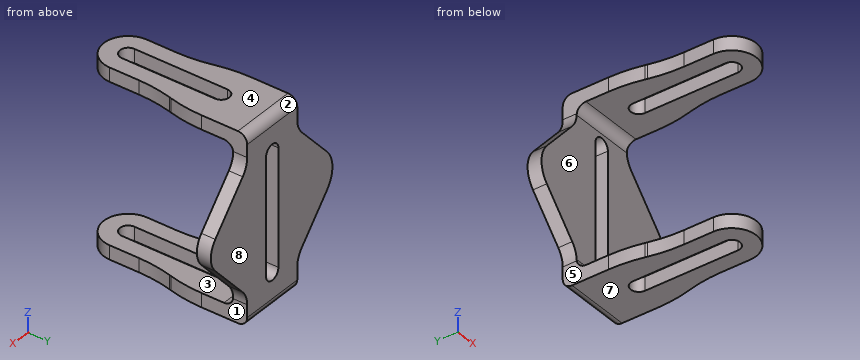
Autodesk Inventor part; units mm, degrees
ref_plane "YZ Plane" through (0, 0, 0) normal (1, 0, 0) x (0, 1, 0)
ref_plane "XZ Plane" through (0, 0, 0) normal (0, 1, 0) x (-1, 0, 0)
ref_plane "XY Plane" through (0, 0, 0) normal (0, 0, 1) x (1, 0, 0)
sketch "Sketch1" plane through (0, 0, 0) normal (0, 1, 0) x (-1, 0, 0)
  line L0 (7.1, -20.1) -> (-7.1, -20.1)
  line L1 (-7.1, -20.1) -> (-7.1, 20.1)
  line L2 (-7.1, 20.1) -> (7.1, 20.1)
  line L3 (7.1, 20.1) -> (7.1, -20.1)
  line L4 (7.1, -20.1) -> (-7.1, 20.1) construction
  line L5 (-7.1, -20.1) -> (7.1, 20.1) construction
  circle A0 centre (0, 12.1) radius 2
  point P0 (0, 0)
  dimension "d0" = 14.2
  dimension "d1" = 40.2
  dimension "d4" = 4
  dimension "d5" = 8
  dimension "d6" = 7.1
extrude "Extrusion1" add sketch "Sketch1" along normal blind 3 contours L0 L1 L2 L3 | A0
sketch "Sketch2" plane through (-7.1, 0, 20.1) normal (0, 0, 1) x (1, 0, 0)
  line L0 (7.1, -28) -> (7.1, -8) construction
  line L1 (8.85, -28) -> (8.85, -8)
  line L2 (5.35, -8) -> (5.35, -28)
  arc A0 (5.35, -28) -> (8.85, -28) centre (7.1, -28) ccw
  arc A1 (8.85, -8) -> (5.35, -8) centre (7.1, -8) ccw
  line L3 (0, 0) -> (0, 3)
  line L4 (0, 0) -> (14.2, 0)
  line L5 (1.85, -28) -> (1.85, -8)
  arc A2 (12.35, -8) -> (1.85, -8) centre (7.1, -8) ccw
  line L6 (12.35, -8) -> (12.35, -28)
  arc A3 (1.85, -28) -> (12.35, -28) centre (7.1, -28) ccw
  line L7 (0, 0) -> (0, -10.5)
  line L8 (0, -10.5) -> (1.85, -18)
  line L9 (14.2, 0) -> (14.2, -10.5)
  line L10 (14.2, -10.5) -> (12.35, -18)
  point P0 (7.1, 0)
  point P1 (7.1, -18)
  point P2 (8.85, -18)
  dimension "d7" = 7.1
  dimension "d8" = 3.5
  dimension "d9" = 20
  dimension "d10" = 18
  dimension "d11" = 3.5
extrude "Extrusion2" add sketch "Sketch2" against normal blind 3
mirror "Mirror1" about plane through (0, 0, 0) normal (0, 0, 1) of "Extrusion2"
fillet "Fillet1" radius 30 8 edges at (7.1, -10.5, 18.6) (5.25, -18, 18.6) (-7.1, -10.5, 18.6) (-5.25, -18, 18.6) (7.1, -10.5, -18.6) (5.25, -18, -18.6) (-7.1, -10.5, -18.6) (-5.25, -18, -18.6)
sketch "Sketch3" plane through (0, 3, 0) normal (0, 1, 0) x (1, 0, 0)
  line L0 (-7.1, -13.5) -> (7.1, -13.5)
  line L1 (-7.1, -13.5) -> (-19.1, 0)
  line L2 (7.1, 13.5) -> (-7.1, 13.5)
  line L3 (-19.1, 0) -> (-7.1, 13.5)
  line L4 (-7.1, 13.5) -> (-7.1, -13.5)
  line L5 (-7.1, 20.1) -> (-7.1, -20.1)
  line L6 (-7.1, 0) -> (-19.1, 0)
  point P0 (0, 0)
  point P1 (-7.1, 0)
  point P2 (-7.1, 14.5)
  point P3 (-7.1, -14.5)
  dimension "d17" = 12
extrude "Extrusion3" add sketch "Sketch3" against normal blind 3
fillet "Fillet4" radius 6 1 edges at (-19.1, 1.5, 0)
fillet "Fillet5" radius 5 2 edges at (-7.1, 1.5, 13.5) (-7.1, 1.5, -13.5)
mirror "Mirror2" about plane through (0, 0, 0) normal (1, 0, 0) of "Extrusion3"
fillet "Fillet6" radius 5 2 edges at (7.1, 1.5, 13.5) (7.1, 1.5, -13.5)
fillet "Fillet7" radius 5 1 edges at (19.1, 1.5, 0)
fillet "Fillet8" radius 2 4 edges at (0, 3, 20.1) (0, 3, -20.1) (0, 0, -17.1) (0, 0, 17.1)
sketch "Sketch4" plane through (0, 3, 0) normal (0, 1, 0) x (1, 0, 0)
  line L0 (0, -12.5) -> (0, 12.5) construction
  line L1 (1.75, -12.5) -> (1.75, 12.5)
  line L2 (-1.75, 12.5) -> (-1.75, -12.5)
  arc A0 (-1.75, -12.5) -> (1.75, -12.5) centre (0, -12.5) ccw
  arc A1 (1.75, 12.5) -> (-1.75, 12.5) centre (0, 12.5) ccw
  point P0 (0, 0)
  dimension "d26" = 3.5
  dimension "d27" = 25
extrude "Extrusion4" cut sketch "Sketch4" against normal blind 10
properties part number "SoporteSensorDeInterrupcionesEJEX"
Could you check a few things on this model? Use its own coordinates, in mm. Face numbers are marked on the shaded views. A direction names the side the tool comes from. Give positions to 0.01 mm unless a question says otherwise; leave off trailing zeros. Order: outer loops, then holes, each group sorted by start corner. A loop starts at its lowest first (then second) coordinate and runs counter-clockwise, first axis right, second up. Notation, with made-up numbers: (60.25, -7.5) -> (85.25, -7.5) arc R9 cw to (85.25, 1.5) -> close; hole circle Ø5 at (-5, 57.25). An arc over 180 degrees is marked (long way). Answer in a Markdown table with one row per item. Add a question column.
Item 1: Imagine slicing it at A-A (x = 0). List the corners of the cut face in (y, z) for me.
Item 2: For the marked faces 1, 2, 3, 4 and 5, which set-ups out of +Z, -Z, +X, -X, +Y, -Y let a thin tool reach every point of the face, with its end or its side?
Item 3: Imagine slicing it at C-C (y = -20.5). List the corners of the cut face in (x, z) for me.
Item 4: Please list where these lines run through material, in increasing order: probe 1 along Z at (x, y) = (6, -7.5); probe 2 along Y at (x, z) = (-6, -14.5); probe 3 along X at (y, z) = (-25, 18.5).
Item 5: I'm going to push flat-ended pins straight in: P1, Ø3.5, axis at y = 2, z = -6, coming from the +X side; P2, Ø3, axis at y = -20, z = -15, coming from the -X side; P3, Ø3.5, axis at y = -15, z = -18.5, coming from the +X side; P4, Ø5, axis at y = -3.5, z = 18, coming from the +X side. Where does each tip first touch, or does it pass through?
Item 6: Imagine slicing it at B-B (z = 5). List the corners of the cut face in (x, y) for me.
Item 7: We'd pull the mould along Z, two halves only. Please class the marked faces 6, 7 and 8: pulls with the +Z half, pulls with the -Z half, needs draft (parallel to the pull), parting line crosses it, or undercut.
Item 8: Imagine slicing it at D-D (y = -1). List the corners of the cut face in (x, z) for me.
Result:
| question | item | result |
|---|---|---|
| 1 | outline | (-33.25, -20.1) -> (-29.75, -20.1) -> (-29.75, -17.1) -> (-33.25, -17.1) -> close; (-33.25, 17.1) -> (-29.75, 17.1) -> (-29.75, 20.1) -> (-33.25, 20.1) -> close; (-6.25, -20.1) -> (1, -20.1) arc R2 ccw to (3, -18.1) -> (3, -14.25) -> (0, -14.25) -> (0, -15.1) arc R2 cw to (-2, -17.1) -> (-6.25, -17.1) -> close; (-6.25, 17.1) -> (-2, 17.1) arc R2 cw to (0, 15.1) -> (0, 14.25) -> (3, 14.25) -> (3, 18.1) arc R2 ccw to (1, 20.1) -> (-6.25, 20.1) -> close |
| 2 | face 1 | -Z, +X, +Y, -Y |
| 2 | face 2 | +Z, +X, -X, +Y |
| 2 | face 3 | +X, -X, -Y |
| 2 | face 4 | +Z, +X, -X, +Y, -Y |
| 2 | face 5 | -Z, -X, +Y, -Y |
| 3 | outline | (-5.27, -20.1) -> (-1.75, -20.1) -> (-1.75, -17.1) -> (-5.27, -17.1) -> close; (-5.27, 17.1) -> (-1.75, 17.1) -> (-1.75, 20.1) -> (-5.27, 20.1) -> close; (1.75, -20.1) -> (5.27, -20.1) -> (5.27, -17.1) -> (1.75, -17.1) -> close; (1.75, 17.1) -> (5.27, 17.1) -> (5.27, 20.1) -> (1.75, 20.1) -> close |
| 4 | probe 1 | -20.1 to -17.1, 17.1 to 20.1 |
| 4 | probe 2 | 0 to 3 |
| 4 | probe 3 | -5.25 to -1.75, 1.75 to 5.25 |
| 5 | P1 | x = 15.32 |
| 5 | P2 | through |
| 5 | P3 | x = 6.41 |
| 5 | P4 | x = 7.1 |
| 6 | outline | (-14.66, 0) -> (-1.75, 0) -> (-1.75, 3) -> (-14.66, 3) -> close; (1.75, 0) -> (14.66, 0) -> (14.66, 3) -> (1.75, 3) -> close |
| 7 | face 6 | undercut |
| 7 | face 7 | pulls with the -Z half |
| 7 | face 8 | needs draft |
| 8 | outline | (-7.1, -20.1) -> (7.1, -20.1) -> (7.1, -16.83) -> (-7.1, -16.83) -> close; (-7.1, 16.83) -> (7.1, 16.83) -> (7.1, 20.1) -> (-7.1, 20.1) -> close |
